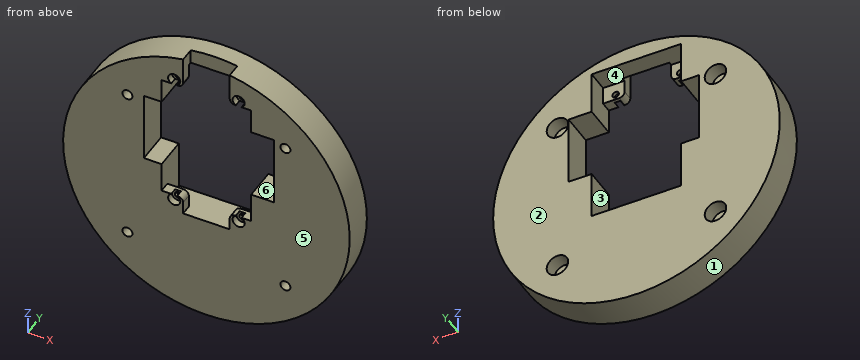
```python
from build123d import *

# Parameters (mm, degrees)
SKETCH1_R                = 40
BOSS_EXTRUDE1_DEPTH      = 8
BOSS_EXTRUDE1_DEPTH_BACK = 1
SKETCH2_W                = 25
SKETCH2_H                = 45.5
CUT_EXTRUDE1_DEPTH       = 6
CUT_EXTRUDE2_DEPTH       = 6
SKETCH4_R                = 3
CUT_EXTRUDE3_DEPTH       = 4
SKETCH5_R                = 1.4
CUT_EXTRUDE4_DEPTH       = 5
CIRPATTERN1_COUNT        = 4
FILLET1_R                = 1.5
SKETCH6_W                = 13
SKETCH6_H                = 8.686825583
CUT_EXTRUDE5_DEPTH       = 4
CUT_EXTRUDE6_START       = -9
SKETCH7_W                = 36.377301766
SKETCH7_H                = 20
CUT_EXTRUDE6_DEPTH       = 9
SKETCH8_R                = 0.9
CUT_EXTRUDE7_DEPTH       = 4
SKETCH9_R                = 1.7
CUT_EXTRUDE10_DEPTH      = 2


with BuildPart() as part:
    # Sketch1 → Boss-Extrude1 (new body, two sides)
    with BuildSketch(Plane(origin=(0, 0, 0), x_dir=(1, 0, 0), z_dir=(0, 1, 0))) as boss_extrude1_sk:
        Circle(SKETCH1_R)
    extrude(amount=BOSS_EXTRUDE1_DEPTH)
    extrude(boss_extrude1_sk.sketch, amount=-BOSS_EXTRUDE1_DEPTH_BACK)

    # Sketch2 → Cut-Extrude1 (cut)
    with BuildSketch(Plane(origin=(0, 8, 0), x_dir=(1, 0, 0), z_dir=(0, 1, 0))):
        with Locations((0, -12.75)):
            Rectangle(SKETCH2_W, SKETCH2_H)
    extrude(amount=-CUT_EXTRUDE1_DEPTH, mode=Mode.SUBTRACT)

    # Sketch3 → Cut-Extrude2 (cut)
    with BuildSketch(Plane(origin=(0, 2, 0), x_dir=(1, 0, 0), z_dir=(0, 1, 0))):
        Polygon((-12.5, 5), (-6.5, 5), (-6.5, 10), (6.5, 10), (6.5, 5), (12.5, 5), (12.5, -30.5), (6.5, -30.5), (6.5, -35.5), (-6.5, -35.5), (-6.5, -30.5), (-12.5, -30.5), align=None)
    extrude(amount=-CUT_EXTRUDE2_DEPTH, mode=Mode.SUBTRACT)

    # Sketch4 → Cut-Extrude3 (cut)
    with BuildSketch(Plane(origin=(0, 8, 0), x_dir=(1, 0, 0), z_dir=(0, 1, 0))):
        with Locations((22.051187962, -22.051187962)):
            Circle(SKETCH4_R)
    cut_extrude3 = extrude(amount=-CUT_EXTRUDE3_DEPTH, mode=Mode.SUBTRACT)

    # Sketch5 → Cut-Extrude4 (cut)
    with BuildSketch(Plane(origin=(0, 4, 0), x_dir=(1, 0, 0), z_dir=(0, 1, 0))):
        with Locations((22.051187962, -22.051187962)):
            Circle(SKETCH5_R)
    cut_extrude4 = extrude(amount=-CUT_EXTRUDE4_DEPTH, mode=Mode.SUBTRACT)

    # CirPattern1: Cut-Extrude3, Cut-Extrude4 ×4 about axis
    cirpattern1_axis = Axis((0, 0, 0), (0, 1, 0))
    for i in range(1, CIRPATTERN1_COUNT):
        add(cut_extrude3.rotate(cirpattern1_axis, i * 360 / CIRPATTERN1_COUNT), mode=Mode.SUBTRACT)
        add(cut_extrude4.rotate(cirpattern1_axis, i * 360 / CIRPATTERN1_COUNT), mode=Mode.SUBTRACT)

    # Fillet1
    fillet1_edges = [part.edges().sort_by_distance(p)[0] for p in [
        (-6.5, 0.5, -5),
        (6.5, 0.5, -5),
        (6.5, 0.5, 30.5),
        (-6.5, 0.5, 30.5),
    ]]
    fillet(fillet1_edges, radius=FILLET1_R)

    # Sketch6 → Cut-Extrude5 (cut)
    with BuildSketch(Plane.XZ.offset(1)):
        with Locations((0, 39.843412792)):
            Rectangle(SKETCH6_W, SKETCH6_H)
    extrude(amount=-CUT_EXTRUDE5_DEPTH, mode=Mode.SUBTRACT)

    # Sketch7 → Cut-Extrude6 (cut)
    with BuildSketch(Plane.XZ.offset(1).offset(CUT_EXTRUDE6_START)):
        with Locations((0.741230287, 13.5)):
            Rectangle(SKETCH7_W, SKETCH7_H)
    extrude(amount=CUT_EXTRUDE6_DEPTH, mode=Mode.SUBTRACT)

    # Sketch8 → Cut-Extrude7 (cut)
    with BuildSketch(Plane(origin=(0, 2, 0), x_dir=(1, 0, 0), z_dir=(0, 1, 0))):
        with Locations((9, -32)):
            Circle(SKETCH8_R)
        with Locations((-9, -32)):
            Circle(SKETCH8_R)
        with Locations((-9, 6.5)):
            Circle(SKETCH8_R)
        with Locations((9, 6.5)):
            Circle(SKETCH8_R)
    extrude(amount=-CUT_EXTRUDE7_DEPTH, mode=Mode.SUBTRACT)

    # Sketch9 → Cut-Extrude10 (cut)
    with BuildSketch(Plane.XZ.offset(1)):
        with Locations((-9, -6.5)):
            Circle(SKETCH9_R)
        with Locations((9, -6.5)):
            Circle(SKETCH9_R)
        with Locations((9, 32)):
            Circle(SKETCH9_R)
        with Locations((-9, 32)):
            Circle(SKETCH9_R)
    extrude(amount=-CUT_EXTRUDE10_DEPTH, mode=Mode.SUBTRACT)


solid = part.part
```
Geometry: final body of the model. Coordinates: model frame, mm. Face numbers are marked on the shaded views. A direction names the side the tool comes from. Round coordinates to 2 decimals unless told otherwise and drop trailing zeros. Write each loop counter-clockwise with the first axis right and the second up, starting at its lowest first coordinate (ties: lowest second). Pieces come first, ordered by that corner, then holes.
Item 1: Material intervals for L1, parallel to Z at x = 22, y = 0; L2, parallel to X at y = 4.25, z = 21.5; L3, parallel to Z at x = 9, y = 1.6, sorted ascending.
Item 2: Mould query, pull axis X, two halves, no side actions, for the marked faces 1, 2 and 3. Classes: +X half, -X half, draft (parallel to the pull), parting line (faces both ways), or undercut.
Item 3: Set-up query: the marked faces 4, 5 and 6. Return all of +Z, -Z, +X, -X, +Y, -Y with unobstructed straight access to the full face (end or side cutting, diameter ignored); none if empty.
Item 4: Section query C-C (y = 6.5). Return loops of the section in (x, z), plus the area to 3 significant figures.
Item 5: Section query B-B (z = 0). Return loops of the section in (x, y), plus the area to 3 significant figures.
Item 6: Pin query (flat end, axial travel): P1, Ø3, axis at x = -21, z = 22, coming from the +Y side; P2, Ø2.5, axis at x = -9.5, z = 33, coming from the +Y side; P3, Ø3.5, axis at y = 1, z = -9, coming from the +X side. Return the tip coordinate at first contact, or that it passes through.
Item 7: Section query D-D (z = -12). Return loops of the section in (x, y).
Item 8: Section query A-A (x = 0). Return loops of the section in (y, z).
Completed:
1. L1: z = -33.41 to -23.45, -20.65 to 20.65, 23.45 to 33.41
1. L2: x = -33.73 to -25, -19.1 to -17.45, 18.93 to 19.1, 25 to 33.73
1. L3: z = -38.97 to -7.4, -5.6 to -5, 30.5 to 31.1, 32.9 to 38.97
2. face 1: parting line
2. face 2: draft
2. face 3: undercut
3. face 4: +Y
3. face 5: +Z, -Z, +X, -X, -Y
3. face 6: +Y, -Y
4. outline: circle Ø80 at (0, 0); hole circle Ø6 at (-22.05, -22.05); hole circle Ø6 at (-22.05, 22.05); hole (-17.45, 3.5) - (-12.5, 3.5) - (-12.5, -10) - (12.5, -10) - (12.5, 3.5) - (18.93, 3.5) - (18.93, 23.5) - (12.5, 23.5) - (12.5, 35.5) - (-12.5, 35.5) - (-12.5, 23.5) - (-17.45, 23.5) - close; hole circle Ø6 at (22.05, -22.05); hole circle Ø6 at (22.05, 22.05)
4. area: 3,550 mm2
5. outline: (-40, -1) - (-12.5, -1) - (-12.5, 8) - (-40, 8) - close; (12.5, -1) - (40, -1) - (40, 8) - (12.5, 8) - close
5. area: 495 mm2
6. P1: stops at y = 4
6. P2: stops at y = 2
6. P3: stops at x = 39.34
7. outline: (-38.16, -1) - (38.16, -1) - (38.16, 8) - (-38.16, 8) - close
8. outline: (-1, -40) - (8, -40) - (8, -10) - (-1, -10) - close; (3, 35.5) - (8, 35.5) - (8, 40) - (3, 40) - close
